from build123d import *

# Parameters (mm, degrees)
SKETCH4_R          = 4.7625
CUT_EXTRUDE2_DEPTH = 114.707959264
CIRPATTERN1_COUNT  = 8
SKETCH6_R          = 40
SKETCH6_R_2        = 31.5
CUT_EXTRUDE3_DEPTH = 10
SKETCH7_W          = 10
SKETCH7_H          = 10.050043706
CUT_EXTRUDE4_DEPTH = 10
CIRPATTERN2_COUNT  = 3
SKETCH9_R          = 2
CUT_EXTRUDE5_DEPTH = 10
CIRPATTERN3_COUNT  = 8


with BuildPart() as part:
    # Sketch3 → Revolve1 (revolve)
    with BuildSketch(Plane(origin=(0, 0, 0), x_dir=(0, 0, -1), z_dir=(1, 0, 0))):
        with BuildLine():
            Line((76.5, 15), (55, 15))
            Line((55, 15), (55, 35))
            Line((55, 35), (22.025, 35))
            Line((22.025, 35), (22.025, 17.36))
            Line((22.025, 17.36), (14.665, 10))
            Line((14.665, 10), (14.665, 0))
            Line((14.665, 0), (19.665, 0))
            ThreePointArc((19.665, 0), (40.232841234, 6.880454009), (53.85, -10))
            Line((53.85, -10), (76.5, -10))
            Line((76.5, -10), (76.5, 15))
        make_face()
    revolve(axis=Axis((0, 0, 0), (0, 1, 0)))

    # Sketch4 → Cut-Extrude2 (cut, symmetric)
    with BuildSketch(Plane(origin=(0, 0, 0), x_dir=(1, 0, 0), z_dir=(0, 1, 0))):
        with Locations(Location((-65.2, 0, 0), (0, 0, 270))):
            Circle(SKETCH4_R)
    cut_extrude2 = extrude(amount=CUT_EXTRUDE2_DEPTH, both=True, mode=Mode.SUBTRACT)

    # CirPattern1: Cut-Extrude2 ×8 about axis
    cirpattern1_axis = Axis((0, 0, 0), (0, 1, 0))
    for i in range(1, CIRPATTERN1_COUNT):
        add(cut_extrude2.rotate(cirpattern1_axis, i * 360 / CIRPATTERN1_COUNT), mode=Mode.SUBTRACT)

    # Sketch6 → Cut-Extrude3 (cut)
    with BuildSketch(Plane(origin=(0, 35, 0), x_dir=(1, 0, 0), z_dir=(0, 1, 0))):
        with Locations(Location((0, 0, 0), (0, 0, 270))):
            Circle(SKETCH6_R)
        with Locations(Location((0, 0, 0), (0, 0, 270))):
            Circle(SKETCH6_R_2, mode=Mode.SUBTRACT)
    extrude(amount=-CUT_EXTRUDE3_DEPTH, mode=Mode.SUBTRACT)

    # Sketch7 → Cut-Extrude4 (cut)
    with BuildSketch(Plane(origin=(0, 35, 0), x_dir=(1, 0, 0), z_dir=(0, 1, 0))):
        with Locations((0, 26.474978147)):
            Rectangle(SKETCH7_W, SKETCH7_H)
    cut_extrude4 = extrude(amount=-CUT_EXTRUDE4_DEPTH, mode=Mode.SUBTRACT)

    # CirPattern2: Cut-Extrude4 ×3 about axis
    cirpattern2_axis = Axis((0, 0, 0), (0, 1, 0))
    for i in range(1, CIRPATTERN2_COUNT):
        add(cut_extrude4.rotate(cirpattern2_axis, i * 360 / CIRPATTERN2_COUNT), mode=Mode.SUBTRACT)

    # Sketch9 → Cut-Extrude5 (cut)
    with BuildSketch(Plane(origin=(0, 35, 0), x_dir=(1, 0, 0), z_dir=(0, 1, 0))):
        with Locations(Location((45.270097093, 18.751488186, 0), (0, 0, 270))):
            Circle(SKETCH9_R)
    cut_extrude5 = extrude(amount=-CUT_EXTRUDE5_DEPTH, mode=Mode.SUBTRACT)

    # CirPattern3: Cut-Extrude5 ×8 about axis
    cirpattern3_axis = Axis((0, 0, 0), (0, 1, 0))
    for i in range(1, CIRPATTERN3_COUNT):
        add(cut_extrude5.rotate(cirpattern3_axis, i * 360 / CIRPATTERN3_COUNT), mode=Mode.SUBTRACT)


solid = part.part
Geometry: final body of the model. Coordinates: model frame, mm. A direction names the side the tool comes from. Round coordinates to 2 decimals unless told otherwise and drop trailing zeros. Loops run counter-clockwise (first coordinate to the right, second up) from the corner with the lowest first, then second, coordinate; pieces in that order, holes last.
Q1. Section A-A on x = 0. State how many separate pieces and enclosed holes the cut face has, plus the area to 3 significant figures.
Q2. Section D-D on x = 65.2. Return loops of the section in (y, z).
Q3. Pin query (flat end, axial travel): P1, Ø4, axis at x = 18.5, y = 8.5, coming from the -Z side; P2, Ø8, axis at y = 23.5, z = 41, coming from the -X side; P3, Ø11, axis at x = 65.2, z = 0, coming from the +Y side. Return the tip coordinate at first contact, or that it passes through.
Q4. Section C-C on z = -65.2. Return loops of the section in (x, y).
Q5. Access query for faces 5 (the cylindrical face through (-27.08, 30.07, -16.09)), 6 (the cylindrical face through (1.03, 2.68, -69.85)). Directions: +Z, -Z, +X, -X, +Y, -Y. A direction counts if a zero-diameter tool reaches every point of the face in a straight line with its end or side. Return the directions, or none.
Q6. Material intervals for L1, parallel to X at y = 32.5, z = 0 (3 decimals); L2, parallel to X at y = 30.5, z = -34; L3, parallel to Z at x = 43, y = 11.5, sorted ascending.
Q7. Pull-direction query (Z, two-part tool) for faces 1 (the cylindrical face through (27.473, 30.07, -15.41)), 2 (the flat face through (-46, -10, -29)), 3 (the conical face through (9.141, 10.357, 11.921)), 4 (the cylindrical face through (53.692, 25.14, 11.923)); classes: released by +Z, released by -Z, zero draft, split by the parting line, or undercut.
Evaluation:
1. separate pieces: 4
1. enclosed holes: 0
1. area: 2,570 mm2
2. outline: (-10, -40.02) - (15, -40.02) - (15, -4.76) - (-10, -4.76) - close; (-10, 4.76) - (15, 4.76) - (15, 40.02) - (-10, 40.02) - close
3. P1: stops at z = -74.7
3. P2: stops at x = -40.69
3. P3: stops at y = 15
4. outline: (-40.02, -10) - (-4.76, -10) - (-4.76, 15) - (-40.02, 15) - close; (4.76, -10) - (40.02, -10) - (40.02, 15) - (4.76, 15) - close
5. face 5: +Y
5. face 6: +Y, -Y
6. L1: x = -55 to -40, -31.5 to -22.025, 22.025 to 31.5, 40 to 55
6. L2: x = -43.23 to -21.07, 21.07 to 43.23
6. L3: z = -63.27 to -49.72, -42.49 to 42.49, 49.72 to 63.27
7. face 1: undercut
7. face 2: zero draft
7. face 3: undercut
7. face 4: split by the parting line
